from build123d import *

# Parameters (mm, degrees)
BOSS_EXTRUDE2_DEPTH = 508
SKETCH5_R           = 38.1
CUT_EXTRUDE1_DEPTH  = 127
SKETCH7_R           = 40.852227979
SKETCH7_R_2         = 38.702110717
CUT_EXTRUDE2_DEPTH  = 127


with BuildPart() as part:
    # Sketch1 → Boss-Extrude2 (new body)
    with BuildSketch(Plane(origin=(0, 0, 0), x_dir=(1, 0, 0), z_dir=(0, 1, 0))):
        Polygon((-464.437614836, 50.8), (424.562385164, 50.8), (500.762385164, -50.8), (-464.437614836, -50.8), align=None)
    extrude(amount=BOSS_EXTRUDE2_DEPTH)

    # Sketch5 → Cut-Extrude1 (cut)
    with BuildSketch(Plane(origin=(0, 508, 0), x_dir=(1, 0, 0), z_dir=(0, 1, 0))):
        with Locations(Location((-235.837614836, 0, 0), (0, 0, 270))):
            Circle(SKETCH5_R)
        with Locations(Location((272.162385164, 0, 0), (0, 0, 270))):
            Circle(SKETCH5_R)
    extrude(amount=-CUT_EXTRUDE1_DEPTH, mode=Mode.SUBTRACT)

    # Sketch7 → Cut-Extrude2 (cut)
    with BuildSketch(Plane.XZ):
        with Locations(Location((-235.837614836, 0, 0), (0, 0, 270))):
            Circle(SKETCH7_R)
        with Locations(Location((272.162385164, 0, 0), (0, 0, 270))):
            Circle(SKETCH7_R_2)
    extrude(amount=-CUT_EXTRUDE2_DEPTH, mode=Mode.SUBTRACT)


solid = part.part
Input: part model. Units: mm. Frame: model coordinates. A direction names the side the tool comes from. Coordinates: 2 decimals unless noted, no trailing zeros. Loops run counter-clockwise (first coordinate to the right, second up) from the corner with the lowest first, then second, coordinate; pieces in that order, holes last.
Q1. Contact query for flat-ended pins moving along their axis: pin 1 (3 mm diameter, centred on y = 328.5, z = 32, fed in from +X); pin 2 (3 mm diameter, centred on y = 109.5, z = 7, fed in from +X); pin 3 (24.5 mm diameter, centred on x = -235, z = 5, fed in from -Y). Output: stop coordinate, or through.
Q2. Cut plane D-D (y = 82.5). Output: boundary loops of the cut face in (x, z), then the cut area to 3 significant figures.
Q3. Material intervals for line 1 (X direction, y = 474.5, z = 15); line 2 (X direction, y = 423, z = -9); line 3 (Y direction, x = -219.5, z = -16), sorted ascending.
Q4. Cut plane C-C (y = 170.5). Output: boundary loops of the cut face in (x, z), then the cut area to 3 significant figures.
Q5. Cut plane A-A (z = 1.5). Output: boundary loops of the cut face in (x, y), then the cut area to 3 significant figures.
Q6. Cut plane B-B (x = -207.5). Output: boundary loops of the cut face in (y, z).
Q7. Draft query along X for faces 4 (the face through (-26, 250, -50.8)), 5 (the face through (462.13, 250.44, -0.71)), 6 (the face through (-464.438, 250, 1)), 7 (the face through (-235, 127, 1)). Return one class per face: +X half, -X half, draft (parallel to the pull), parting line (faces both ways), or undercut.
Q8. Set-up query: faces 1 (the face through (-235, 381, -1)), 2 (the face through (273, 127, 1)), 3 (the face through (25, 508, -1)). Return all of +Z, -Z, +X, -X, +Y, -Y with unobstructed straight access to the full face (end or side cutting, diameter ignored); none if empty.
Working result:
1. pin 1: stops at x = 487.79
1. pin 2: stops at x = 469.04
1. pin 3: stops at y = 127
2. outline: (-464.44, -50.8) - (424.56, -50.8) - (500.76, 50.8) - (-464.44, 50.8) - close; hole circle Ø81.7 at (-235.84, 0); hole circle Ø77.4 at (272.16, 0)
2. area: 84,200 mm2
3. line 1: x = -464.44 to -270.86, -200.81 to 237.14, 307.19 to 473.91
3. line 2: x = -464.44 to -272.86, -198.82 to 235.14, 309.18 to 455.91
3. line 3: y = 127 to 381
4. outline: (-464.44, -50.8) - (424.56, -50.8) - (500.76, 50.8) - (-464.44, 50.8) - close
4. area: 94,200 mm2
5. outline: (-464.44, 0) - (-276.66, 0) - (-276.66, 127) - (-195.01, 127) - (-195.01, 0) - (233.49, 0) - (233.49, 127) - (310.84, 127) - (310.84, 0) - (463.79, 0) - (463.79, 508) - (310.23, 508) - (310.23, 381) - (234.09, 381) - (234.09, 508) - (-197.77, 508) - (-197.77, 381) - (-273.91, 381) - (-273.91, 508) - (-464.44, 508) - close
5. area: 432,000 mm2
6. outline: (0, -50.8) - (508, -50.8) - (508, -25.47) - (381, -25.47) - (381, 25.47) - (508, 25.47) - (508, 50.8) - (0, 50.8) - (0, 29.43) - (127, 29.43) - (127, -29.43) - (0, -29.43) - close
7. face 4: draft
7. face 5: +X half
7. face 6: -X half
7. face 7: undercut
8. face 1: +Y
8. face 2: -Y
8. face 3: +Z, -Z, +X, -X, +Y
